Autodesk Inventor part; units mm, degrees
ref_plane "YZ Plane" through (0, 0, 0) normal (1, 0, 0) x (0, 1, 0)
ref_plane "XZ Plane" through (0, 0, 0) normal (0, 1, 0) x (-1, 0, 0)
ref_plane "XY Plane" through (0, 0, 0) normal (0, 0, 1) x (1, 0, 0)
sketch "Sketch1" plane through (0, 0, 0) normal (0, 1, 0) x (-1, 0, 0)
  line L0 (0, 0) -> (-54.66, 0)
  line L1 (-54.66, 0) -> (-54.66, -82.94)
  line L2 (-54.66, -82.94) -> (0, -82.94)
  line L3 (0, -82.94) -> (0, 0)
  dimension "d0" = 54.66
  dimension "d1" = 82.94
extrude "Extrusion1" add sketch "Sketch1" along normal blind 2.3
sketch "Sketch2" plane through (0, 2.3, 0) normal (0, 1, 0) x (1, 0, 0)
  point P0 (0, 0)
sketch "Sketch3" plane through (0, 2.3, 0) normal (0, 1, 0) x (1, 0, 0)
  line L0 (2.85, 7.15) -> (51.81, 7.15)
  line L1 (51.81, 7.15) -> (51.81, 80.59)
  line L2 (51.81, 80.59) -> (2.85, 80.59)
  line L3 (2.85, 80.59) -> (2.85, 7.15)
  line L4 (54.66, 82.94) -> (0, 82.94)
  line L5 (0, 82.94) -> (0, 0)
  line L6 (0, 0) -> (54.66, 0)
  line L7 (54.66, 0) -> (54.66, 82.94)
  line L8 (54.66, 82.94) -> (0, 82.94)
  line L9 (0, 82.94) -> (0, 0)
  dimension "d4" = 73.44
  dimension "d5" = 48.96
  dimension "d6" = 2.35
  dimension "d7" = 2.85
extrude "Extrusion2" add sketch "Sketch3" along normal blind 1
sketch "Sketch4" plane through (0, 3.3, 0) normal (0, 1, 0) x (1, 0, 0)
  line L0 (-1.52, -1.5) -> (56.18, -1.5)
  line L1 (56.18, -1.5) -> (56.18, 89.1)
  line L2 (56.18, 89.1) -> (-1.52, 89.1)
  line L3 (-1.52, 89.1) -> (-1.52, -1.5)
  line L4 (0, 0) -> (54.66, 0)
  line L5 (54.66, 82.94) -> (0, 82.94)
  line L6 (2.85, 7.15) -> (51.81, 7.15)
  line L7 (51.81, 80.59) -> (2.85, 80.59)
  line L8 (51.81, 7.15) -> (2.85, 7.15)
  line L9 (2.85, 7.15) -> (2.85, 80.59)
  line L10 (2.85, 80.59) -> (51.81, 80.59)
  line L11 (51.81, 80.59) -> (51.81, 7.15)
  point P0 (27.33, 82.94)
  point P1 (27.33, 89.1)
  dimension "d10" = 90.6
  dimension "d11" = 57.7
  dimension "d12" = 1.5
extrude "Extrusion3" add sketch "Sketch4" along normal blind 0.7
fillet "Fillet1" radius 1 4 edges at (-1.52, 3.65, 1.5) (56.18, 3.65, 1.5) (56.18, 3.65, -89.1) (-1.52, 3.65, -89.1)
sketch "Sketch5" plane through (0, 2.3, 0) normal (0, 1, 0) x (1, 0, 0)
  line L0 (51.81, 7.15) -> (2.85, 7.15)
  line L1 (2.85, 80.59) -> (51.81, 80.59)
  line L2 (2.85, 7.15) -> (51.81, 7.15)
  line L3 (51.81, 7.15) -> (51.81, 80.59)
  line L4 (51.81, 80.59) -> (2.85, 80.59)
  line L5 (2.85, 80.59) -> (2.85, 7.15)
  point P0 (0, 0)
extrude "Extrusion4" add sketch "Sketch5" along normal blind 1.6999
properties part number "LCD+Cover"
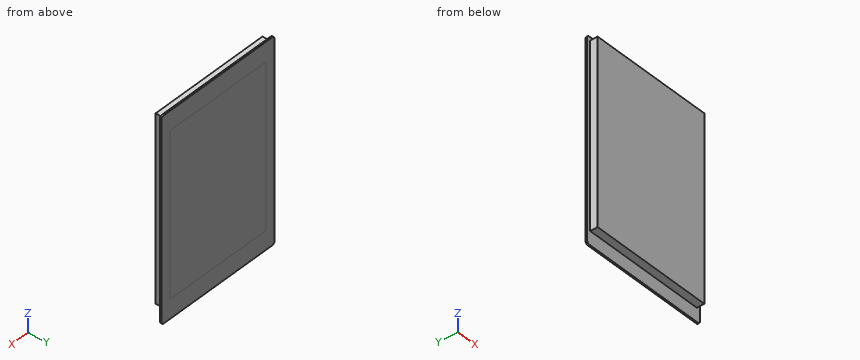
Part model, mm, in its own coordinate system. Give positions to 0.01 mm unless a question says otherwise; leave off trailing zeros. Write each loop counter-clockwise with the first axis right and the second up, starting at its lowest first coordinate (ties: lowest second). Pieces come first, ordered by that corner, then holes. Notation, with made-up numbers: (35, 77.25) -> (58, 77.25) arc R26 ccw to (58, 100.25) -> close; hole circle Ø10 at (-27.75, -14.5). An arc over 180 degrees is marked (long way). Put each result on its own line as item: value. Start each with the question number.
Item 1: Pin check, flat tips, straight feed: pin 1 Ø5 at (x, z) = (45.5, -35.5) entering from -Y; pin 2 Ø1.6 at (y, z) = (1.5, -36) entering from +X. Stop position of each tip, or through.
Item 2: Wall check: L1, parallel to Z at x = 48, y = 2.65; L2, parallel to X at y = 0.4, z = -6. Give the ranges that are in metal, low to high. Write a range as [from, to].
Item 3: Cut at C-C (y = 1.4). List the corners of the cut face in (x, z).
Answer list:
1. pin 1: stops at y = 0
1. pin 2: stops at x = 54.66
2. L1: z = [-82.94, 0]
2. L2: x = [0, 54.66]
3. outline: (0, -82.94) -> (54.66, -82.94) -> (54.66, 0) -> (0, 0) -> close
